Drawing for the job (mm, zero at the part's lowest x, y, z). Coordinates: 2 decimals unless noted, no trailing zeros. Loops run counter-clockwise (first coordinate to the right, second up) from the corner with the lowest first, then second, coordinate; pieces in that order, holes last. Notation, with made-up numbers: (61, -15.75) - (96, -15.75) arc R10 ccw to (96, -1.75) - close; hole circle Ø1 at (4, 87.25). An arc over 180 degrees is marked (long way). One line per item, written item: value.
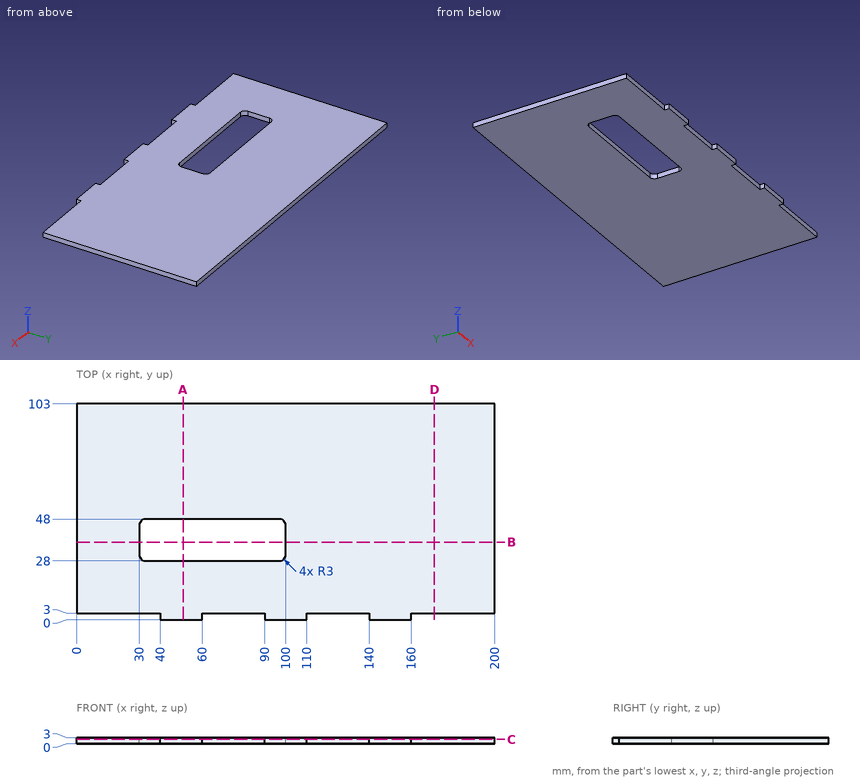
Item 1: Cut at C-C, the plane z = 2.15. Write the cut outline in (x, y).
Check result:
outline: (0, 3) - (40, 3) - (40, 0) - (60, 0) - (60, 3) - (90, 3) - (90, 0) - (110, 0) - (110, 3) - (140, 3) - (140, 0) - (160, 0) - (160, 3) - (200, 3) - (200, 103) - (0, 103) - close; hole (30, 31) arc R3 ccw to (33, 28) - (97, 28) arc R3 ccw to (100, 31) - (100, 45) arc R3 ccw to (97, 48) - (33, 48) arc R3 ccw to (30, 45) - close
Item 2: Cut at B-B, the plane y = 37. Write the cut outline in (x, z), then the cut area to 3 significant figures.
Check result:
outline: (0, 0) - (30, 0) - (30, 3) - (0, 3) - close; (100, 0) - (200, 0) - (200, 3) - (100, 3) - close
area: 390 mm^2
Item 3: Cut at A-A, the plane x = 51. Write the cut outline in (y, z), then the cut area to 3 significant figures.
Check result:
outline: (0, 0) - (28, 0) - (28, 3) - (0, 3) - close; (48, 0) - (103, 0) - (103, 3) - (48, 3) - close
area: 249 mm^2
Item 4: Drop flat-ended pins along their axis: P1, Ø0.9, axis at x = 68, z = 1, coming from the -Y side; P2, Ø0.9, axis at y = 1, z = 1, coming from the -X side; P3, Ø0.9, axis at y = 1.5, z = 1, coming from the +X side. Give the stop position or say it passes through.
Check result:
P1: stops at y = 3
P2: stops at x = 40
P3: stops at x = 160
Item 5: Cut at D-D, the plane x = 171. Write the cut outline in (y, z).
Check result:
outline: (3, 0) - (103, 0) - (103, 3) - (3, 3) - close
Item 6: Probe probe 1 along X at (y, z) = (34.5, 2); probe 2 along Y at (x, z) = (69, 1.7); probe 3 along Y at (x, z) = (169, 2.95). List the from-to ranges inside material, lowest first. Write a range as from..to.
Check result:
probe 1: x = 0..30, 100..200
probe 2: y = 3..28, 48..103
probe 3: y = 3..103
